Verification items for the finished model (mm, model axes). A direction names the side the tool comes from. Coordinates: 2 decimals unless noted, no trailing zeros. Write each loop counter-clockwise with the first axis right and the second up, starting at its lowest first coordinate (ties: lowest second). Pieces come first, ordered by that corner, then holes. Notation, with made-up numbers: (-10.5, 73.5) -> (17.5, 73.5) arc R11 cw to (17.5, 84.5) -> close; hole circle Ø6 at (23, 72). An arc over 180 degrees is marked (long way). Use a Markdown table: item, result. Add a question column.
from build123d import *

# Parameters (mm, degrees)
SKETCH_2_R          = 1.6
EXTRUDE_2_DEPTH     = 3
SKETCH_3_W          = 48
SKETCH_3_H          = 8
EXTRUDE_3_DEPTH     = 2
SKETCH_4_W          = 16
SKETCH_4_H          = 8
EXTRUDE_4_DEPTH     = 45
CUT_EXTRUDE_1_DEPTH = 59.966091951
CUT_EXTRUDE_2_DEPTH = 5


with BuildPart() as part:
    # 草图2 → 凸台-拉伸2 (new body)
    with BuildSketch(Plane(origin=(0, 0, 0), x_dir=(1, 0, 0), z_dir=(0, 1, 0))):
        Polygon((-28, 36), (-10, 36), (-10, 29.949747468), (-3.450252532, 23.4), (3.450252532, 23.4), (10, 29.949747468), (10, 36), (28, 36), (28, 0), (-28, 0), align=None)
        with Locations(Location((-10, 25, 0), (0, 0, 270))):
            Circle(SKETCH_2_R, mode=Mode.SUBTRACT)
        with Locations(Location((10, 25, 0), (0, 0, 270))):
            Circle(SKETCH_2_R, mode=Mode.SUBTRACT)
    extrude(amount=-EXTRUDE_2_DEPTH)

    # 草图3 → 凸台-拉伸3 (add)
    with BuildSketch(Plane(origin=(0, 0, 0), x_dir=(1, 0, 0), z_dir=(0, 1, 0))):
        with Locations((0, 18)):
            Rectangle(SKETCH_3_W, SKETCH_3_H)
    extrude(amount=EXTRUDE_3_DEPTH)

    # 草图4 → 凸台-拉伸4 (add)
    with BuildSketch(Plane(origin=(0, 2, 0), x_dir=(1, 0, 0), z_dir=(0, 1, 0))):
        with Locations((0, 18)):
            Rectangle(SKETCH_4_W, SKETCH_4_H)
    extrude(amount=EXTRUDE_4_DEPTH)

    # 草图5 → 切除-拉伸1 (cut, through all)
    with BuildSketch(Plane.XY.offset(-14)):
        with BuildLine():
            Line((2.5, 39), (2.5, 19))
            ThreePointArc((2.5, 19), (0, 16.5), (-2.5, 19))
            Line((-2.5, 19), (-2.5, 39))
            ThreePointArc((-2.5, 39), (0, 41.5), (2.5, 39))
        make_face()
    extrude(amount=-CUT_EXTRUDE_1_DEPTH, mode=Mode.SUBTRACT)

    # 草图6 → 切除-拉伸2 (cut)
    with BuildSketch(Plane.XY.offset(-14)):
        with BuildLine():
            Line((4.5, 40), (4.5, 18))
            ThreePointArc((4.5, 18), (0, 13.5), (-4.5, 18))
            Line((-4.5, 18), (-4.5, 40))
            ThreePointArc((-4.5, 40), (0, 44.5), (4.5, 40))
        make_face()
    extrude(amount=-CUT_EXTRUDE_2_DEPTH, mode=Mode.SUBTRACT)


solid = part.part
1) Cross-section at D-D on z = -25. Record the boundary of the cut face in (x, y), then the cut area to 3 significant figures.
2) Cross-section at C-C on x = -20. Record the boundary of the cut face in (y, z), then the cut area to 3 significant figures.
3) Cross-section at B-B on y = 24. Record the boundary of the cut face in (x, z).
4) Set-up check for faces 4 (the face through (4.5, 29, -16)), 5 (the face through (-0.1, 41.5, -20.5)), 6 (the face through (16, 2, -18)), 7 (the face through (-8, 24, -18)), 8 (the face through (0, -1, -23.4)): record each of +Z, -Z, +X, -X, +Y, -Y from which the full face is reachable in a straight line by a thin tool's end or side.
5) Release check for a two-part mould opening along Y. For faces 1 (the face through (0.4, 0, -22.3)), 2 (the face through (0.1, 16.5, -20.5)), 3 (the face through (28, -1, -18)) record: released by +Y, released by -Y, zero draft, split by the parting line, or undercut.
6) Cross-section at A-A on x = 0. Record the boundary of the cut face in (y, z), then the cut area to 3 significant figures.
7) Gauge pin test, flat ends, axial feed: pin 1 (1.5 mm diameter, centred on y = 33, z = -21, fed in from -X); pin 2 (6 mm diameter, centred on x = -17.5, z = -16, fed in from +Y); pin 3 (2.5 mm diameter, centred on y = 26, z = -16, fed in from +X); pin 4 (1.9 mm diameter, centred on x = 10, z = -25, fed in from +Y). Record the tip position at first contact, or that the pin passes through.
8) Thickness scan on L1, parallel to X at y = 28, z = -16; L2, parallel to X at y = -1.8, z = -25; L3, parallel to Z at x = -2, y = 13.5. Record the ranges inside material, lowest first.
Returned:
| question | item | result |
|---|---|---|
| 1 | outline | (-28, -3) -> (-11.6, -3) -> (-11.6, 0) -> (-28, 0) -> close; (-8.4, -3) -> (-5.05, -3) -> (-5.05, 0) -> (-8.4, 0) -> close; (5.05, -3) -> (8.4, -3) -> (8.4, 0) -> (5.05, 0) -> close; (11.6, -3) -> (28, -3) -> (28, 0) -> (11.6, 0) -> close |
| 1 | area | 118 mm² |
| 2 | outline | (-3, -36) -> (0, -36) -> (0, -22) -> (2, -22) -> (2, -14) -> (0, -14) -> (0, 0) -> (-3, 0) -> close |
| 2 | area | 124 mm² |
| 3 | outline | (-8, -22) -> (-2.5, -22) -> (-2.5, -19) -> (-4.5, -19) -> (-4.5, -14) -> (-8, -14) -> close; (2.5, -22) -> (8, -22) -> (8, -14) -> (4.5, -14) -> (4.5, -19) -> (2.5, -19) -> close |
| 4 | face 4 | +Z |
| 4 | face 5 | +Z, -Z |
| 4 | face 6 | +Z, -Z, +X, +Y |
| 4 | face 7 | +Z, -Z, -X, +Y |
| 4 | face 8 | -Z, +Y, -Y |
| 5 | face 1 | released by +Y |
| 5 | face 2 | undercut |
| 5 | face 3 | zero draft |
| 6 | outline | (-3, -23.4) -> (0, -23.4) -> (0, -22) -> (16.5, -22) -> (16.5, -19) -> (13.5, -19) -> (13.5, -14) -> (0, -14) -> (0, 0) -> (-3, 0) -> close; (41.5, -22) -> (47, -22) -> (47, -14) -> (44.5, -14) -> (44.5, -19) -> (41.5, -19) -> close |
| 6 | area | 216 mm² |
| 7 | pin 1 | stops at x = -8 |
| 7 | pin 2 | stops at y = 2 |
| 7 | pin 3 | stops at x = 8 |
| 7 | pin 4 | passes through |
| 8 | L1 | x = -8 to -4.5, 4.5 to 8 |
| 8 | L2 | x = -28 to -11.6, -8.4 to -5.05, 5.05 to 8.4, 11.6 to 28 |
| 8 | L3 | z = -22 to -14 |
